For this review, use the dimensioned drawing (mm, ordinates from the lowest corner) and the shaded views. A direction names the side the tool comes from. Coordinates: 2 decimals unless noted, no trailing zeros. Write each loop counter-clockwise with the first axis right and the second up, starting at its lowest first coordinate (ties: lowest second). Pieces come first, ordered by that corner, then holes. Notation, with made-up numbers: (5, 89) - (20, 89) arc R22 cw to (20, 103) - close; hole circle Ø5 at (35, -12). An arc over 180 degrees is marked (long way). One line per item, written item: value.
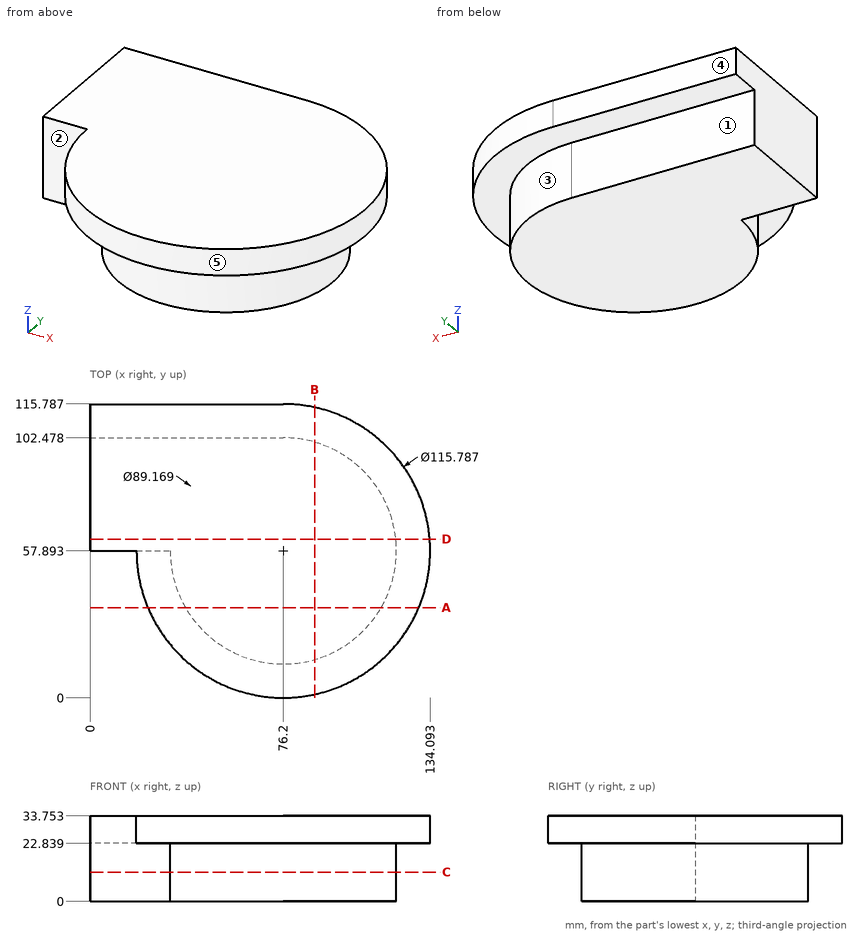
1. Consider section C-C, the plane z = 11.5. Write out the cut boundary in (x, y) (1 decimal).
Answer block:
outline: (0, 57.9) - (31.6, 57.9) arc R44.6 ccw (long way) to (76.2, 102.5) - (0, 102.5) - close
2. Insertion check: pin 1 Ø10 at (y, z) = (46.5, 8) entering from +X; pin 2 Ø7 at (x, z) = (40.5, 7.5) entering from +Y; pin 3 Ø8 at (y, z) = (26, 4.5) entering from -X. Each pin has a flat end and moves straight along its axis. Give the tip position at first contact, or say it passes through.
Answer block:
pin 1: stops at x = 120.32
pin 2: stops at y = 102.48
pin 3: stops at x = 41.42
3. Consider section A-A, the plane y = 35.5. Write out the cut boundary in (x, z), then the cut area to 3 significant figures.
Answer block:
outline: (22.81, 22.84) - (37.65, 22.84) - (37.65, 0) - (114.75, 0) - (114.75, 22.84) - (129.59, 22.84) - (129.59, 33.75) - (22.81, 33.75) - close
area: 2,930 mm^2
4. Consider section D-D, the plane y = 62.5. Write out the cut boundary in (x, z), then the cut area to 3 significant figures.
Answer block:
outline: (0, 0) - (120.55, 0) - (120.55, 22.84) - (133.91, 22.84) - (133.91, 33.75) - (0, 33.75) - close
area: 4,210 mm^2
5. Consider section B-B, the plane x = 88.5. Write out the cut boundary in (y, z) (1 decimal).
Answer block:
outline: (1.3, 22.8) - (15, 22.8) - (15, 0) - (100.7, 0) - (100.7, 22.8) - (114.5, 22.8) - (114.5, 33.8) - (1.3, 33.8) - close
6. Wall thickness on line 1 along Z through (x, y) = (36, 32); line 2 along X through (y, z) = (59, 30); line 3 along Y through (x, z) = (9, 22.5): over which ranges is each line inside the solid? List them lowest first.
Answer block:
line 1: z = 22.84 to 33.75
line 2: x = 0 to 134.08
line 3: y = 57.89 to 102.48
7. For the marked faces 1, 2, 3, 4 and 5, list the 3-axis set-ups (+Z, -Z, +X, -X, +Y, -Y) from which the entire face can be reached by the end or side of a thin tool; tool diameter is ignored.
Answer block:
face 1: -Z, +X, -X, +Y
face 2: -Z, -X, -Y
face 3: -Z
face 4: +Z, -Z, +X, -X, +Y
face 5: +Z, -Z
